Solid Edge part; units mm, degrees
sketch "Sketch1" plane through (0, 0, 0) normal (0, 0, 1) x (1, 0, 0)
  circle A0 centre (0, 0) radius 1.5
extrude "Protrusion1" add sketch "Sketch1" along normal blind 5
sketch "Sketch2" plane through (0, 0, 5) normal (0, 0, 1) x (1, 0, 0)
  line L0 (2.25, 1.299) -> (0, 2.5981)
  line L1 (0, 2.5981) -> (-2.25, 1.299)
  line L2 (-2.25, 1.299) -> (-2.25, -1.299)
  line L3 (-2.25, -1.299) -> (0, -2.5981)
  line L4 (0, -2.5981) -> (2.25, -1.299)
  line L5 (2.25, -1.299) -> (2.25, 1.299)
extrude "ExtrudedProtrusion_2" add sketch "Sketch2" along normal blind 39.9
sketch "Sketch3" plane through (0, 0, 44.9) normal (0, 0, 1) x (0, 1, 0)
  circle A0 centre (0, 0) radius 1.5
extrude "ExtrudedCutout_1" cut sketch "Sketch3" against normal blind 10
fillet "Round_1" radius 0.2 20 edges at (2.25, -1.299, 24.95) (2.25, 1.299, 24.95) (2.25, 0, 44.9) (1.125, 1.9486, 44.9) (0, -1.5, 44.9) (0, 2.5981, 24.95) (1.125, 1.9486, 5) (2.25, 0, 5) (1.125, -1.9486, 5) (0, -2.5981, 24.95) (1.125, -1.9486, 44.9) (-1.125, -1.9486, 44.9) (-1.125, -1.9486, 5) (-2.25, -1.299, 24.95) (-2.25, 0, 44.9) (-1.125, 1.9486, 44.9) (-2.25, 1.299, 24.95) (-2.25, 0, 5) (-1.125, 1.9486, 5) (-1.5, 0, 0)
properties material "Brass, yellow brass"
Model file for the job. Use its own axes, mm. A direction names the side the tool comes from. Coordinates: 2 decimals unless noted, no trailing zeros. Loops run counter-clockwise (first coordinate to the right, second up) from the corner with the lowest first, then second, coordinate; pieces in that order, holes last. Notation, with made-up numbers: (66.25, 2.5) - (73.25, 2.5) arc R21 ccw to (73.25, 37.5) - close; hole circle Ø8 at (82.25, 70). An arc over 180 degrees is marked (long way). Answer as a JSON object with one key per item and string values. Group by question number.
(1) Probe line 1 along X through (y, z) = (0, 38.25); line 2 along Z through (x, y) = (-0.45, 0.5); line 3 along Y through (x, z) = (0, 37.25). List the from-to ranges inside material, lowest first.
(2) Cut at A-A (y = 0). Give the cut face in (x, z), then the cut area to 3 significant figures.
(3) Tool access for faces 1 (the face through (0, -2, 5)), 2 (the face through (0, -2, 44.9)), 3 (the face through (0, 0, 34.9)): list every direction of +Z, -Z, +X, -X, +Y, -Y with a clear straight run to the whole face (end or side of a thin tool).
(4) Flat gauge pins, fed straight in: pin 1 (1.5 mm diameter, centred on x = 0.5, y = -0.5, fed in from +Z); pin 2 (1 mm diameter, centred on x = 1.5, z = 10, fed in from -Y). Where does each tip first touch, or does it go through?
(5) Cut at B-B (z = 6). Give the cut face in (x, y).
(6) Two-plate mould, pull along X, no slides. Class faces 4 (the face through (-0.07, -1.5, 39.87)), 5 (the face through (-1.081, -1.905, 44.843)), 6 (the face through (1.11, -1.89, 5.06)): released by +X, released by -X, zero draft, split by the parting line, or undercut.
Geometry says:
{
 "1": {"line 1": "x = -2.25 to -1.5, 1.5 to 2.25", "line 2": "z = 0 to 34.9", "line 3": "y = -2.57 to -1.5, 1.5 to 2.57"},
 "2": {"outline": "(-2.25, 5.2) arc R0.2 ccw to (-2.05, 5) - (-1.5, 5) - (-1.5, 0.2) arc R0.2 ccw to (-1.3, 0) - (1.3, 0) arc R0.2 ccw to (1.5, 0.2) - (1.5, 5) - (2.05, 5) arc R0.2 ccw to (2.25, 5.2) - (2.25, 44.7) arc R0.2 ccw to (2.05, 44.9) - (1.7, 44.9) arc R0.2 ccw to (1.5, 44.7) - (1.5, 34.9) - (-1.5, 34.9) - (-1.5, 44.7) arc R0.2 ccw to (-1.7, 44.9) - (-2.05, 44.9) arc R0.2 ccw to (-2.25, 44.7) - close", "area": "164 mm^2"},
 "3": {"face 1": "-Z", "face 2": "+Z, +X, -X, +Y, -Y", "face 3": "+Z"},
 "4": {"pin 1": "stops at z = 34.9", "pin 2": "stops at y = -2.02"},
 "5": {"outline": "(-2.25, -1.18) arc R0.2 ccw to (-2.15, -1.36) - (-0.1, -2.54) arc R0.2 ccw to (0.1, -2.54) - (2.15, -1.36) arc R0.2 ccw to (2.25, -1.18) - (2.25, 1.18) arc R0.2 ccw to (2.15, 1.36) - (0.1, 2.54) arc R0.2 ccw to (-0.1, 2.54) - (-2.15, 1.36) arc R0.2 ccw to (-2.25, 1.18) - close"},
 "6": {"face 4": "undercut", "face 5": "released by -X", "face 6": "released by +X"}
}
